The listing builds one solid part. Answer for the finished solid, in the listing's coordinates (mm). Give positions to 0.01 mm unless a question says otherwise; leave off trailing zeros. Write each loop counter-clockwise with the first axis right and the second up, starting at its lowest first coordinate (ties: lowest second). Pieces come first, ordered by that corner, then holes. Notation, with made-up numbers: (14.5, 47) - (47.5, 47) arc R14 cw to (47.5, 53) - close; hole circle Ø1 at (-38, 8). An arc over 180 degrees is marked (long way). Write each question's results on one line, items separated by ' | '. Start each with the question number.
Q1. Section D-D (y = -3) is taken. Determine the outline of the cut face in (x, z) (3 decimals).
Q2. Section A-A (x = 0) is taken. Determine the outline of the cut face in (y, z) (3 decimals), plus the area to 3 significant figures.
Q3. Flat-ended cylindrical pins translate along their axes: pin 1 Ø2 at (x, z) = (0, 1.5) entering from +Y; pin 2 Ø1 at (x, y) = (0, 2.5) entering from -Z; pin 3 Ø1 at (x, z) = (-2, 3) entering from -Y. Find the tip coordinate at first contact, or state that the pin passes through.
Q4. Find the intervals of material crossed by probe 1 along X at (y, z) = (3.25, 0.55) (3 decimals); probe 2 along Z at (x, y) = (-0.5, -1.25); probe 3 along Z at (x, y) = (1.5, -2), in increasing order.
Q5. For a pull along Y with two mould halves and no side action, classify faces 1 (the face through (0.31, 1.39, 3.05)), 2 (the face through (0, 0, 0.12)), 3 (the face through (-1.44, 0.74, 2.7)) as pulls with the +Y half, pulls with the -Y half, needs draft (parallel to the pull), parting line crosses it, or undercut.
Q6. Section C-C (z = 0.55) is taken. Determine the outline of the cut face in (x, y) (3 decimals).
```python
from build123d import *

# Parameters (mm, degrees)
SKIZZE1_W                                  = 6.3
SKIZZE1_H                                  = 6.3
AUFSATZ_LINEAR_AUSTRAGEN1_DEPTH            = 2.7
SKIZZE2_R                                  = 1.425
AUFSATZ_LINEAR_AUSTRAGEN2_DEPTH            = 3.4
FL_CHE_VERSCHIEBEN1_BY                     = 0.12
SKIZZE3_W                                  = 0.75
SKIZZE3_H                                  = 1.61
AUFSATZ_LINEAR_AUSTRAGEN3_DEPTH            = 1.3
SPIEGELN1_AT_THE_SECOND_PLANE_COPY_1_SKE_W = 0.75
SPIEGELN1_AT_THE_SECOND_PLANE_COPY_1_SKE_H = 1.61
SPIEGELN1_AT_THE_SECOND_PLANE_COPY_1_DEPTH = 1.3


with BuildPart() as part:
    # Skizze1 → Aufsatz-Linear austragen1 (new body)
    with BuildSketch(Plane.XY):
        Rectangle(SKIZZE1_W, SKIZZE1_H)
    extrude(amount=AUFSATZ_LINEAR_AUSTRAGEN1_DEPTH)

    # Skizze2 → Aufsatz-Linear austragen2 (add)
    with BuildSketch(Plane.XY):
        with Locations(Location((0, 0, 0), (0, 0, 180))):
            Circle(SKIZZE2_R)
    extrude(amount=AUFSATZ_LINEAR_AUSTRAGEN2_DEPTH)

    # Fläche verschieben1: a face moved inward by 0.12
    extrude(part.faces().sort_by_distance((0, 0, 0))[0], amount=FL_CHE_VERSCHIEBEN1_BY, dir=(0, 0, 1), mode=Mode.SUBTRACT)

    # Skizze3 → Aufsatz-Linear austragen3 (add)
    with BuildSketch(Plane.XY):
        with Locations((-2, 2.705)):
            Rectangle(SKIZZE3_W, SKIZZE3_H)
    aufsatz_linear_austragen3 = extrude(amount=AUFSATZ_LINEAR_AUSTRAGEN3_DEPTH)

    # Spiegeln1: Aufsatz-Linear austragen3 across plane
    add(aufsatz_linear_austragen3.mirror(Plane.ZX))

    # Spiegeln1 at the second plane: Aufsatz-Linear austragen3 across plane
    add(aufsatz_linear_austragen3.mirror(Plane(origin=(0, 0, 0), x_dir=(0, 0, 1), z_dir=(1, 0, 0))))

    # Spiegeln1 at the second plane copy 1 ske → Spiegeln1 at the second plane copy 1 (add)
    with BuildSketch(Plane(origin=(0, 0, 0), x_dir=(-1, 0, 0), z_dir=(0, 0, 1))):
        with Locations((-2, 2.705)):
            Rectangle(SPIEGELN1_AT_THE_SECOND_PLANE_COPY_1_SKE_W, SPIEGELN1_AT_THE_SECOND_PLANE_COPY_1_SKE_H)
    extrude(amount=SPIEGELN1_AT_THE_SECOND_PLANE_COPY_1_DEPTH)


solid = part.part
```
Answers below:
1) outline: (-3.15, 0.12) - (-2.375, 0.12) - (-2.375, 0) - (-1.625, 0) - (-1.625, 0.12) - (1.625, 0.12) - (1.625, 0) - (2.375, 0) - (2.375, 0.12) - (3.15, 0.12) - (3.15, 2.7) - (-3.15, 2.7) - close
2) outline: (-3.15, 0.12) - (3.15, 0.12) - (3.15, 2.7) - (1.425, 2.7) - (1.425, 3.4) - (-1.425, 3.4) - (-1.425, 2.7) - (-3.15, 2.7) - close | area: 18.2 mm2
3) pin 1: stops at y = 3.15 | pin 2: stops at z = 0.12 | pin 3: stops at y = -3.15
4) probe 1: x = -2.375 to -1.625, 1.625 to 2.375 | probe 2: z = 0.12 to 3.4 | probe 3: z = 0.12 to 2.7
5) face 1: parting line crosses it | face 2: undercut | face 3: needs draft
6) outline: (-3.15, -3.15) - (-2.375, -3.15) - (-2.375, -3.51) - (-1.625, -3.51) - (-1.625, -3.15) - (1.625, -3.15) - (1.625, -3.51) - (2.375, -3.51) - (2.375, -3.15) - (3.15, -3.15) - (3.15, 3.15) - (2.375, 3.15) - (2.375, 3.51) - (1.625, 3.51) - (1.625, 3.15) - (-1.625, 3.15) - (-1.625, 3.51) - (-2.375, 3.51) - (-2.375, 3.15) - (-3.15, 3.15) - close
